Build history of the part. All positions in model axes, mm. A direction names the side the tool comes from. Give positions to 0.01 mm unless a question says otherwise; leave off trailing zeros. Write each loop counter-clockwise with the first axis right and the second up, starting at its lowest first coordinate (ties: lowest second). Pieces come first, ordered by that corner, then holes. Notation, with made-up numbers: (-14.75, -4) -> (-2.75, -4) arc R22 cw to (-2.75, 29) -> close; hole circle Ø7 at (81, -38.75). An arc over 180 degrees is marked (long way). Put each result on its own line as item: value.
Autodesk Inventor part; units mm, degrees
ref_plane "YZ Plane" through (0, 0, 0) normal (1, 0, 0) x (0, 1, 0)
ref_plane "XZ Plane" through (0, 0, 0) normal (0, 1, 0) x (-1, 0, 0)
ref_plane "XY Plane" through (0, 0, 0) normal (0, 0, 1) x (1, 0, 0)
ref_plane "Work Plane1" through (0, 0, 0) normal (0, 0, 1) x (1, 0, 0)
sketch "Sketch1" plane through (0, 0, 0) normal (0, 0, 1) x (1, 0, 0)
  line L0 (39.878985, 283.001047) -> (46.807188, 279.001047)
  line L1 (118.687297, 237.501047) -> (-32.001123, 324.501047)
  line L2 (118.687297, 237.501047) -> (112.687297, 227.108743)
  line L3 (-38.001123, 314.108743) -> (112.687297, 227.108743)
  line L4 (-32.001123, 324.501047) -> (-38.001123, 314.108743)
  line L5 (40.807188, 268.608743) -> (46.807188, 279.001047)
  line L6 (33.878985, 272.608743) -> (39.878985, 283.001047)
  line L7 (40.807188, 268.608743) -> (33.878985, 272.608743)
  circle A0 centre (68.259454, 214.654052) radius 27.5 construction
  line L8 (52.931544, 261.608743) -> (21.754629, 279.608743)
  line L9 (21.754629, 279.608743) -> (15.754629, 269.216438)
  line L10 (15.754629, 269.216438) -> (46.931544, 251.216438)
  line L11 (46.931544, 251.216438) -> (52.931544, 261.608743)
  point P0 (0, 0)
  dimension "d0" = 55
  dimension "d1" = 12
  dimension "d2" = 14
  dimension "d3" = 14
sketch "Sketch1 outline for Extrusion1" plane through (0, 0, 0) normal (0, 0, 1) x (1, 0, 0)
  line L0 (15.754629, 269.216438) -> (46.931544, 251.216438)
  line L1 (21.754629, 279.608743) -> (15.754629, 269.216438)
  line L2 (52.931544, 261.608743) -> (21.754629, 279.608743)
  line L3 (46.931544, 251.216438) -> (52.931544, 261.608743)
extrude "Extrusion1" add sketch "Sketch1 outline for Extrusion1" along normal blind 10
fillet "Fillet1" radius 6 2 edges at (15.7546, 269.2164, 5) (46.9315, 251.2164, 5)
sketch "Sketch2" plane through (0, 0, 10) normal (0, 0, 1) x (1, 0, 0)
  arc A0 (18.754629, 274.41259) -> (20.950782, 266.216438) centre (23.950782, 271.41259) ccw
  arc A1 (41.735391, 254.216438) -> (49.931544, 256.41259) centre (44.735391, 259.41259) ccw
  point P0 (0, 0)
hole "Hole1" at (23.950782, 271.41259, 10) at (44.735391, 259.41259, 10) direction (0, 0, -1) diameter 3.5 end through all countersink diameter 8 countersink angle 90
sketch "Sketch3" plane through (0, 0, 10) normal (0, 0, 1) x (1, 0, 0)
  line L0 (52.931544, 261.608743) -> (21.754629, 279.608743)
  line L1 (42.539239, 267.608743) -> (32.146934, 273.608743)
  line L2 (32.146934, 273.608743) -> (26.146934, 263.216438)
  line L3 (26.146934, 263.216438) -> (36.539239, 257.216438)
  line L4 (36.539239, 257.216438) -> (42.539239, 267.608743)
  line L5 (21.754629, 279.608743) -> (18.754629, 274.41259)
  line L6 (49.931544, 256.41259) -> (52.931544, 261.608743)
  point P0 (0, 0)
  dimension "d14" = 12
  dimension "d15" = 12
  dimension "d16" = 12
sketch "Sketch3 outline for Extrusion2" plane through (0, 0, 10) normal (0, 0, 1) x (1, 0, 0)
  line L0 (26.146934, 263.216438) -> (36.539239, 257.216438)
  line L1 (32.146934, 273.608743) -> (26.146934, 263.216438)
  line L2 (42.539239, 267.608743) -> (32.146934, 273.608743)
  line L3 (36.539239, 257.216438) -> (42.539239, 267.608743)
extrude "Extrusion2" add sketch "Sketch3 outline for Extrusion2" along normal blind 47
sketch "Sketch4" plane through (21.754629, 279.608743, 10) normal (0.5, 0.8660254, 0) x (0.8660254, -0.5, 0)
  circle A0 centre (18, -41) radius 4
  point P0 (120.96431, 10)
sketch "Sketch4 outline for Extrusion3" plane through (21.754629, 279.608743, 10) normal (0.5, 0.8660254, 0) x (0.8660254, -0.5, 0)
  circle A0 centre (18, -41) radius 4
extrude "Extrusion3" cut sketch "Sketch4 outline for Extrusion3" against normal through all
fillet "Fillet2" radius 6 2 edges at (39.5392, 262.4126, 57) (29.1469, 268.4126, 57)
fillet "Fillet3" radius 1 2 edges at (29.1469, 268.4126, 10) (39.5392, 262.4126, 10)
draft "FaceDraft1" angle 2 pull direction (0, 0, 1) faces at (37.48227, 270.528385, 23.009722) fixed edges at (37.343087, 270.608743, 0)
equation "\"d2\" = d3"
equation "\"d15\" = d16"
properties part number "backcover_clamp"
1) Tool access for faces 4 (the flat face through (20.276, 277.047, 4.93)), 5 (the flat face through (29.092, 268.317, 30.72)), 6 (the flat face through (39.403, 262.176, 30.72)): list every direction of +Z, -Z, +X, -X, +Y, -Y with a clear straight run to the whole face (end or side of a thin tool).
Filled sheet:
face 4: +Z, -Z, -X, +Y
face 5: +Z, -X, +Y
face 6: +Z, +X, -Y
2) Wall check: L1, parallel to Z at x = 28.5, y = 275.25; L2, parallel to X at y = 264.25, z = 51; L3, parallel to X at y = 271.5, z = 6. Give the ranges that are in metal, low to high.
Filled sheet:
L1: 0 to 10
L2: 26.74 to 29.05, 38.29 to 40.6
L3: 17.95 to 22.2, 25.7 to 35.38
3) Slice it at A-A (z = 52). Write the cut outline in (x, y).
Filled sheet:
outline: (26.22, 263.17) -> (27.99, 262.15) -> (33.08, 270.97) -> (31.31, 271.99) -> close; (34.7, 258.28) -> (36.47, 257.26) -> (41.56, 266.08) -> (39.79, 267.1) -> close
4) Pull direction X, two halves, no side cores. Call faces 1 (the flat face through (21.09, 274.43, 10)), 2 (the cylindrical face through (37.57, 262.61, 55.29)), 3 (the cylindrical face through (25.02, 272.8, 3.82)): released by +X, released by -X, zero draft, split by the parting line, or undercut.
Filled sheet:
face 1: zero draft
face 2: released by +X
face 3: undercut
5) Pin check, flat tips, straight feed: pin 1 (4 mm diameter, centred on x = 44.74, y = 259.41, fed in from +Z); pin 2 (6 mm diameter, centred on x = 34.5, y = 272, fed in from +Z); pin 3 (6 mm diameter, centred on x = 24, z = 19, fed in from +Y); pin 4 (2 mm diameter, centred on x = 24, y = 265.5, fed in from -Z). Stop position of each tip, or through.
Filled sheet:
pin 1: z = 8.01
pin 2: z = 56.95
pin 3: y = 264.69
pin 4: z = 0
6) Slice it at B-B (z = 36). Write the cut outline in (x, y).
Filled sheet:
outline: (26.15, 263.22) -> (36.54, 257.22) -> (41.91, 266.52) -> (31.52, 272.52) -> close
7) Slice it at C-C (z = 15). Write the cut outline in (x, y), plus the area to 3 significant figures.
Filled sheet:
outline: (26.15, 263.22) -> (36.54, 257.22) -> (42.28, 267.16) -> (31.89, 273.16) -> close
area: 138 mm2
